Design review of the part built by this model. Coordinates are the model's own, in mm. Face numbers are marked on the shaded views. A direction names the side the tool comes from. Coordinates: 2 decimals unless noted, no trailing zeros. Loops run counter-clockwise (first coordinate to the right, second up) from the corner with the lowest first, then second, coordinate; pieces in that order, holes last.
from build123d import *

# Parameters (mm, degrees)
BASE_DEPTH          = 3
SKETCH2_W           = 57
SKETCH2_H           = 68.2942
SHELL_DEPTH         = 1.5
SKETCH3_R           = 1.375
THROUGH_HOLES_DEPTH = 70.842801106
SKETCH6_R           = 1.375
SKETCH6_R_2         = 2
SOCKET_HOLES_DEPTH  = 0.5
SKETCH7_W           = 8.5
SKETCH7_H           = 8.5
BOSS_EXTRUDE2_DEPTH = 2.8
BOSS_EXTRUDE3_DEPTH = 4.1
SKETCH9_W           = 4.9
SKETCH9_H           = 3.32367647
BOSS_EXTRUDE4_DEPTH = 6.028194003
SKETCH10_W          = 2.805255888
SKETCH10_H          = 4.105255888
BOSS_EXTRUDE5_DEPTH = 6.5752


with BuildPart() as part:
    # Sketch1 → Base (new body)
    with BuildSketch(Plane(origin=(0, 26.414945084, 0), x_dir=(1, 0, 0), z_dir=(0, 1, 0))):
        with BuildLine():
            Line((-4.892059596, -40.449863775), (54.607940404, -40.449863775))
            ThreePointArc((54.607940404, -40.449863775), (56.198930662, -39.790854032), (56.857940404, -38.199863775))
            Line((56.857940404, -38.199863775), (56.857940404, 32.594336225))
            ThreePointArc((56.857940404, 32.594336225), (56.198930662, 34.185326483), (54.607940404, 34.844336225))
            Line((54.607940404, 34.844336225), (-4.892059596, 34.844336225))
            ThreePointArc((-4.892059596, 34.844336225), (-6.483049854, 34.185326483), (-7.142059596, 32.594336225))
            Line((-7.142059596, 32.594336225), (-7.142059596, -38.199863775))
            ThreePointArc((-7.142059596, -38.199863775), (-6.483049854, -39.790854032), (-4.892059596, -40.449863775))
        make_face()
    extrude(amount=BASE_DEPTH)

    # Sketch2 → Shell (cut)
    with BuildSketch(Plane.XZ.offset(-26.414945084)):
        with Locations((24.857940404, 2.802763775)):
            Rectangle(SKETCH2_W, SKETCH2_H)
    extrude(amount=-SHELL_DEPTH, mode=Mode.SUBTRACT)

    # Sketch3 → Through Holes (cut, through all)
    with BuildSketch(Plane(origin=(0, 29.414945084, 0), x_dir=(1, 0, 0), z_dir=(0, 1, 0))):
        with Locations(Location((-5.091807064, 32.794083694, 0), (0, 0, 180))):
            Circle(SKETCH3_R)
        with Locations(Location((54.807687872, 32.794083694, 0), (0, 0, 180))):
            Circle(SKETCH3_R)
        with Locations(Location((43.107940404, 10.094336225, 0), (0, 0, 180))):
            Circle(SKETCH3_R)
        with Locations(Location((36.257940404, -20.199611243, 0), (0, 0, 180))):
            Circle(SKETCH3_R)
        with Locations(Location((54.807687872, -38.399611243, 0), (0, 0, 180))):
            Circle(SKETCH3_R)
        with Locations(Location((-5.091807064, -38.399611243, 0), (0, 0, 180))):
            Circle(SKETCH3_R)
    extrude(amount=-THROUGH_HOLES_DEPTH, mode=Mode.SUBTRACT)

    # Sketch6 → Socket Holes (cut)
    # profile 1 of 6: a face of its own
    with BuildSketch(Plane(origin=(0, 29.414945084, 0), x_dir=(1, 0, 0), z_dir=(0, 1, 0))):
        with BuildLine():
            ThreePointArc((-7.142059596, -38.199863775), (-6.483049854, -39.790854032), (-4.892059596, -40.449863775))
            Line((-4.892059596, -40.449863775), (-3.091807064, -40.449863775))
            Line((-3.091807064, -40.449863775), (-3.091807064, -38.399611243))
            ThreePointArc((-3.091807064, -38.399611243), (-3.677593502, -36.98539768), (-5.091807064, -36.399611243))
            Line((-5.091807064, -36.399611243), (-7.142059596, -36.399611243))
            Line((-7.142059596, -36.399611243), (-7.142059596, -38.199863775))
        make_face()
        with Locations(Location((-5.091807064, -38.399611243, 0), (0, 0, 180))):
            Circle(SKETCH6_R, mode=Mode.SUBTRACT)
    # profile 2 of 6: a face of its own
    with BuildSketch(Plane(origin=(0, 29.414945084, 0), x_dir=(1, 0, 0), z_dir=(0, 1, 0))):
        with Locations(Location((36.257940404, -20.199611243, 0), (0, 0, 180))):
            Circle(SKETCH6_R_2)
        with Locations(Location((36.257940404, -20.199611243, 0), (0, 0, 180))):
            Circle(SKETCH6_R, mode=Mode.SUBTRACT)
    # profile 3 of 6: a face of its own
    with BuildSketch(Plane(origin=(0, 29.414945084, 0), x_dir=(1, 0, 0), z_dir=(0, 1, 0))):
        with BuildLine():
            Line((52.807687872, -38.399611243), (52.807687872, -40.449863775))
            Line((52.807687872, -40.449863775), (54.607940404, -40.449863775))
            ThreePointArc((54.607940404, -40.449863775), (56.198930662, -39.790854032), (56.857940404, -38.199863775))
            Line((56.857940404, -38.199863775), (56.857940404, -36.399611243))
            Line((56.857940404, -36.399611243), (54.807687872, -36.399611243))
            ThreePointArc((54.807687872, -36.399611243), (53.39347431, -36.98539768), (52.807687872, -38.399611243))
        make_face()
        with Locations(Location((54.807687872, -38.399611243, 0), (0, 0, 180))):
            Circle(SKETCH6_R, mode=Mode.SUBTRACT)
    # profile 4 of 6: a face of its own
    with BuildSketch(Plane(origin=(0, 29.414945084, 0), x_dir=(1, 0, 0), z_dir=(0, 1, 0))):
        with Locations(Location((43.107940404, 10.094336225, 0), (0, 0, 180))):
            Circle(SKETCH6_R_2)
        with Locations(Location((43.107940404, 10.094336225, 0), (0, 0, 180))):
            Circle(SKETCH6_R, mode=Mode.SUBTRACT)
    # profile 5 of 6: a face of its own
    with BuildSketch(Plane(origin=(0, 29.414945084, 0), x_dir=(1, 0, 0), z_dir=(0, 1, 0))):
        with BuildLine():
            Line((54.807687872, 30.794083694), (56.857940404, 30.794083694))
            Line((56.857940404, 30.794083694), (56.857940404, 32.594336225))
            ThreePointArc((56.857940404, 32.594336225), (56.198930662, 34.185326483), (54.607940404, 34.844336225))
            Line((54.607940404, 34.844336225), (52.807687872, 34.844336225))
            Line((52.807687872, 34.844336225), (52.807687872, 32.794083694))
            ThreePointArc((52.807687872, 32.794083694), (53.39347431, 31.379870131), (54.807687872, 30.794083694))
        make_face()
        with Locations(Location((54.807687872, 32.794083694, 0), (0, 0, 180))):
            Circle(SKETCH6_R, mode=Mode.SUBTRACT)
    # profile 6 of 6: a face of its own
    with BuildSketch(Plane(origin=(0, 29.414945084, 0), x_dir=(1, 0, 0), z_dir=(0, 1, 0))):
        with BuildLine():
            Line((-7.142059596, 32.594336225), (-7.142059596, 30.794083694))
            Line((-7.142059596, 30.794083694), (-5.091807064, 30.794083694))
            ThreePointArc((-5.091807064, 30.794083694), (-3.677593502, 31.379870131), (-3.091807064, 32.794083694))
            Line((-3.091807064, 32.794083694), (-3.091807064, 34.844336225))
            Line((-3.091807064, 34.844336225), (-4.892059596, 34.844336225))
            ThreePointArc((-4.892059596, 34.844336225), (-6.483049854, 34.185326483), (-7.142059596, 32.594336225))
        make_face()
        with Locations(Location((-5.091807064, 32.794083694, 0), (0, 0, 180))):
            Circle(SKETCH6_R, mode=Mode.SUBTRACT)
    extrude(amount=-SOCKET_HOLES_DEPTH, mode=Mode.SUBTRACT)

    # Sketch7 → Boss-Extrude2 (add)
    with BuildSketch(Plane.XZ.offset(-27.914945084)):
        with Locations((8.757575778, 30.275109563)):
            Rectangle(SKETCH7_W, SKETCH7_H)
    extrude(amount=BOSS_EXTRUDE2_DEPTH)

    # Sketch8 → Boss-Extrude3 (add)
    with BuildSketch(Plane.XZ.offset(-27.914945084)):
        with BuildLine():
            Line((26.274319641, 23.450802906), (26.274319641, 20.79902621))
            ThreePointArc((26.274319641, 20.79902621), (25.981426422, 20.091919429), (25.274319641, 19.79902621))
            Line((25.274319641, 19.79902621), (17.388533203, 19.79902621))
            Line((17.388533203, 19.79902621), (15.974319641, 21.213239773))
            Line((15.974319641, 21.213239773), (15.974319641, 23.450802906))
            Line((15.974319641, 23.450802906), (15.974319641, 26.350802906))
            Line((15.974319641, 26.350802906), (15.974319641, 28.588366038))
            Line((15.974319641, 28.588366038), (17.034979813, 29.64902621))
            Line((17.034979813, 29.64902621), (24.860106079, 29.64902621))
            Line((24.860106079, 29.64902621), (26.274319641, 28.234812648))
            Line((26.274319641, 28.234812648), (26.274319641, 26.350802906))
            Line((26.274319641, 26.350802906), (26.274319641, 23.450802906))
        make_face()
    extrude(amount=BOSS_EXTRUDE3_DEPTH)

    # Sketch9 → Boss-Extrude4 (add)
    with BuildSketch(Plane.XZ.offset(-27.914945084)):
        with Locations((6.478182604, 6.956579663)):
            Rectangle(SKETCH9_W, SKETCH9_H)
    extrude(amount=BOSS_EXTRUDE4_DEPTH)

    # Sketch10 → Boss-Extrude5 (add)
    with BuildSketch(Plane.XZ.offset(-27.914945084)):
        with Locations((17.740823979, 9.706286862)):
            Rectangle(SKETCH10_W, SKETCH10_H)
    extrude(amount=BOSS_EXTRUDE5_DEPTH)


solid = part.part
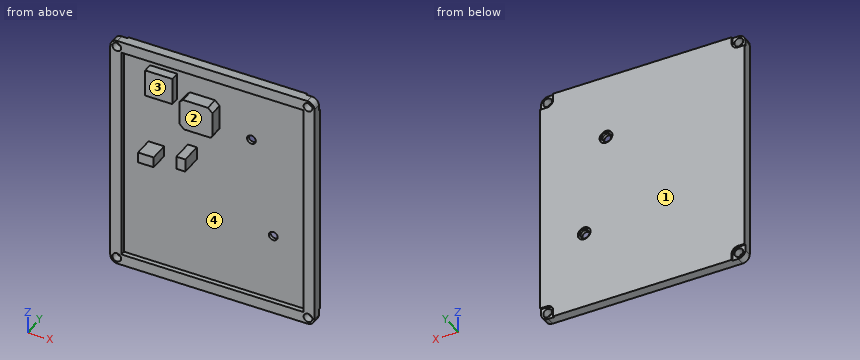
Q1. Take a section at B-B, the plane z = -29. Write out the cut boundary in (x, y), then the cut area to 4 significant figures.
Q2. Machinability: for the marked faces 1 and 2, which of the approach directions +Z, -Z, +X, -X, +Y, -Y give a long, thin tool a straight path to every point of the face, cutting with its end or side? Answer none if there is none.
Q3. Take a section at D-D, the plane x = 36. Write out the cut boundary in (y, z), then the cut area to 3 significant figures.
Q4. Clearance check with flat-ended pins moving along their axes: pin 1 Ø9.5 at (x, z) = (7, 30.5) entering from -Y; pin 2 Ø1 at (x, z) = (8.5, 9.5) entering from -Y; pin 3 Ø3.5 at (x, z) = (-5.09, 38.4) entering from -Y. State where each tip first meets the part, or that it passes through.
Q5. Take a section at C-C, the plane x = 1.5. Write out the cut boundary in (y, z).
Q6. The part is to be moulded in two halves that separate along X. For the marked faces 3 and 4, say which applies: pulls with the +X half, pulls with the -X half, needs draft (parallel to the pull), parting line crosses it, or undercut.
Q7. For line 1 (X direction, y = 26.5, z = -4); line 2 (Z direction, x = 34.5, y = 27); line 3 (Z direction, x = 6, y = 25.25), list the stretches that pass through material, from the lowest coordinate up.
Q8. Take a section at A-A, the plane y = 23. Write out the cut boundary in (x, z), then the cut area to 3 significant figures.
Entries:
1. outline: (-7.14, 26.41) - (-3.64, 26.41) - (-3.64, 27.91) - (53.36, 27.91) - (53.36, 26.41) - (56.86, 26.41) - (56.86, 29.41) - (-7.14, 29.41) - close
1. area: 106.5 mm2
2. face 1: +Z, -Z, +X, -X, +Y
2. face 2: +Z, +X, -X, -Y
3. outline: (26.41, -34.84) - (29.41, -34.84) - (29.41, 18.22) - (28.91, 18.22) - (28.91, 18.85) - (27.91, 18.85) - (27.91, -31.34) - (26.41, -31.34) - close; (26.41, 36.95) - (27.91, 36.95) - (27.91, 21.55) - (28.91, 21.55) - (28.91, 22.18) - (29.41, 22.18) - (29.41, 40.45) - (26.41, 40.45) - close
3. area: 119 mm2
4. pin 1: stops at y = 25.11
4. pin 2: stops at y = 27.91
4. pin 3: stops at y = 26.41
5. outline: (26.41, -34.84) - (29.41, -34.84) - (29.41, 40.45) - (26.41, 40.45) - (26.41, 36.95) - (27.91, 36.95) - (27.91, -31.34) - (26.41, -31.34) - close
6. face 3: needs draft
6. face 4: undercut
7. line 1: x = -7.14 to -3.64, 53.36 to 56.86
7. line 2: z = -34.84 to -31.34, 36.95 to 40.45
7. line 3: z = 5.29 to 8.62, 26.03 to 34.53
8. outline: (4.03, 5.29) - (8.93, 5.29) - (8.93, 8.62) - (4.03, 8.62) - close; (16.34, 7.65) - (19.14, 7.65) - (19.14, 11.76) - (16.34, 11.76) - close
8. area: 27.8 mm2
